```python
from build123d import *

# Parameters (mm, degrees)
SKETCH1_R           = 4.445
EXTRUDE1_DEPTH      = 38.1
SKETCH32_R          = 3.175
CUT_EXTRUDE9_DEPTH  = 39.1
SKETCH34_R          = 3.429
CUT_EXTRUDE11_DEPTH = 1.524
CUT_EXTRUDE11_TAPER = 45
CHAMFER1_SIZE       = 0.254
SKETCH30_R          = 3.175
CUT_EXTRUDE7_DEPTH  = 12.7
CUT_EXTRUDE8_DEPTH  = 12.7


with BuildPart() as part:
    # Sketch1 → Extrude1 (new body)
    with BuildSketch(Plane.XY):
        Circle(SKETCH1_R)
    extrude(amount=-EXTRUDE1_DEPTH)

    # Sketch32 → Cut-Extrude9 (cut, through all)
    with BuildSketch(Plane.XY):
        Circle(SKETCH32_R)
    extrude(amount=-CUT_EXTRUDE9_DEPTH, mode=Mode.SUBTRACT)

    # Sketch34 → Cut-Extrude11 (cut)
    with BuildSketch(Plane.XY):
        Circle(SKETCH34_R)
    extrude(amount=-CUT_EXTRUDE11_DEPTH, taper=CUT_EXTRUDE11_TAPER, mode=Mode.SUBTRACT)

    # Chamfer1
    chamfer1_edges = [part.edges().sort_by_distance(p)[0] for p in [
        (-4.445, 0, 0),
    ]]
    chamfer(chamfer1_edges, length=CHAMFER1_SIZE)

    # Sketch29 → Revolve2 (revolve)
    with BuildSketch(Plane(origin=(0, 0, 0), x_dir=(0, 0, -1), z_dir=(1, 0, 0))):
        with BuildLine():
            Line((16.328571429, 0), (16.328571429, 2.350110803))
            Line((16.328571429, 2.350110803), (16.328571429, 4.445))
            Line((16.328571429, 4.445), (16.630196429, 4.445))
            ThreePointArc((16.630196429, 4.445), (18.413645234, 4.771067643), (19.966347576, 5.707083234))
            ThreePointArc((19.966347576, 5.707083234), (20.815620725, 6.31294757), (21.771428571, 6.731))
            ThreePointArc((21.771428571, 6.731), (29.935714286, 8.001), (38.1, 6.731))
            Line((38.1, 6.731), (38.1, 0))
            Line((38.1, 0), (16.328571429, 0))
        make_face()
    revolve(axis=Axis((0, 0, 0), (0, 0, -1)))

    # Sketch30 → Cut-Extrude7 (cut, symmetric)
    with BuildSketch(Plane(origin=(0, 0, 0), x_dir=(0, 0, -1), z_dir=(1, 0, 0))):
        with Locations((30.842857143, 0)):
            Circle(SKETCH30_R)
        with BuildLine():
            Line((44.45, 8.001), (36.83, 8.001))
            ThreePointArc((36.83, 8.001), (38.1, 0), (36.83, -8.001))
            Line((36.83, -8.001), (44.45, -8.001))
            Line((44.45, -8.001), (44.45, 8.001))
        make_face()
    extrude(amount=CUT_EXTRUDE7_DEPTH, both=True, mode=Mode.SUBTRACT)

    # Sketch31 → Cut-Extrude8 (cut, symmetric)
    with BuildSketch(Plane(origin=(0, 0, 0), x_dir=(1, 0, 0), z_dir=(0, 1, 0))):
        with BuildLine():
            Line((1.778, 38.1), (1.778, 21.771428571))
            ThreePointArc((1.778, 21.771428571), (2.484425862, 18.87551952), (4.445, 16.630196429))
            Line((4.445, 16.630196429), (14.478, 16.630196429))
            Line((14.478, 16.630196429), (14.478, 38.1))
            Line((14.478, 38.1), (1.778, 38.1))
        make_face()
        with BuildLine():
            Line((-1.778, 38.1), (-1.778, 21.771428571))
            ThreePointArc((-1.778, 21.771428571), (-2.484425862, 18.87551952), (-4.445, 16.630196429))
            Line((-4.445, 16.630196429), (-14.478, 16.630196429))
            Line((-14.478, 16.630196429), (-14.478, 38.1))
            Line((-14.478, 38.1), (-1.778, 38.1))
        make_face()
    extrude(amount=CUT_EXTRUDE8_DEPTH, both=True, mode=Mode.SUBTRACT)


solid = part.part
```
Design review of the part built by this model. Coordinates are the model's own, in mm. A direction names the side the tool comes from. Round coordinates to 2 decimals unless told otherwise and drop trailing zeros. Order: outer loops, then holes, each group sorted by start corner. A loop starts at its lowest first (then second) coordinate and runs counter-clockwise, first axis right, second up. Notation, with made-up numbers: (-30.75, -18) - (24.25, -18) arc R22 ccw to (24.25, 12) - close; hole circle Ø1 at (47, 73.25). An arc over 180 degrees is marked (long way). One line per question, with ' | ' between items.
Item 1: Machinability: for faces 4 (the face through (0, 0, -16.329)), 5 (the face through (-2.193, 0.091, -19.524)), 6 (the face through (1.778, -2, -28)), which of the approach directions +Z, -Z, +X, -X, +Y, -Y give a long, thin tool a straight path to every point of the face, cutting with its end or side? Answer none if there is none.
Checks:
face 4: +Z | face 5: -Z, -X, +Y, -Y | face 6: -Z, +X, +Y, -Y
Item 2: Take a section at A-A, the plane z = -10. Write out the cut boundary in (x, y) (3 decimals), then the cut area to 3 significant figures.
Checks:
outline: circle Ø8.89 at (0, 0); hole circle Ø6.35 at (0, 0) | area: 30.4 mm²
Item 3: For P1, Ø4.5, axis at y = 1.5, z = -32.5, coming from the +X side; P2, Ø2, axis at y = 0, z = -25.5, coming from the -X side; P3, Ø3, axis at x = -0.5, y = -1, coming from the +Z side, all flat-tipped, find the tip position at first contact; note any pin that passes through.
Checks:
P1: x = 1.78 | P2: x = -1.78 | P3: z = -16.33
Item 4: Draft analysis for pull direction X (two halves, no side actions). For faces 1 (the face through (-2, -3, 0)), 2 (the face through (-1.778, 2, -28)), 3 (the face through (-2.52, -1.93, -8.18)), state which applies: +X half, -X half, draft (parallel to the pull), parting line (faces both ways), or undercut.
Checks:
face 1: draft | face 2: -X half | face 3: undercut
Item 5: Wall thickness on line 1 (Y direction, x = 0, z = -5) (3 decimals); line 2 (Z direction, x = 0.75, y = -1.5); line 3 (X direction, y = 1.25, z = -3): over which ranges is each line inside the solid? List them lowest first. Write a range as [from, to].
Checks:
line 1: [-4.445, -3.175], [3.175, 4.445] | line 2: [-38.06, -33.64], [-28.04, -16.33] | line 3: [-4.27, -2.92], [2.92, 4.27]
